Could you check a few things on this model? Use its own coordinates, in mm. A direction names the side the tool comes from. Round coordinates to 2 decimals unless told otherwise and drop trailing zeros. Write each loop counter-clockwise with the first axis right and the second up, starting at its lowest first coordinate (ties: lowest second). Pieces come first, ordered by that corner, then holes. Notation, with made-up numbers: (86.5, -38.75) -> (134.5, -38.75) arc R20 ccw to (134.5, -2.75) -> close; hole circle Ø9 at (62, 89). An arc over 180 degrees is marked (long way). Return JSON: item names as keys, results as strings.
from build123d import *

# Parameters (mm, degrees)
BOSS_EXTRUDE1_DEPTH    = 15
M2_5_CLEARANCE_HOLE1_D = 2.9
M2_5_CLEARANCE_HOLE2_D = 2.9
FILLET1_START          = -15
FILLET1_DEPTH          = 30
FILLET1_START_2        = 4.5
FILLET1_2_OUTLINE_R    = 1.45
FILLET1_2_DEPTH        = 2.5
CUT_EXTRUDE1_START     = -4.5
SKETCH6_R              = 2.75
SKETCH6_R_2            = 2.749999999
CUT_EXTRUDE1_DEPTH     = 10


with BuildPart() as part:
    # Sketch1 → Boss-Extrude1 (new, symmetric)
    with BuildSketch(Plane.XY):
        Polygon((0, 0), (0, -10), (4.5, -10), (4.5, -3.267573076), (86.73, 23.5), (96.73, 23.5), (96.73, 28), (86.016016224, 28), align=None)
    extrude(amount=BOSS_EXTRUDE1_DEPTH, both=True)

    # M2.5 Clearance Hole1 (through all)
    with Locations(Plane(origin=(0, 23.5, 0), x_dir=(-1, 0, 0), z_dir=(0, -1, 0))):
        with Locations((-91.73, -6), (-91.73, 6)):
            Hole(M2_5_CLEARANCE_HOLE1_D / 2)

    # M2.5 Clearance Hole2 (through all)
    with Locations(Plane(origin=(4.5, 0, 0), x_dir=(0, 0, -1), z_dir=(1, 0, 0))):
        with Locations((-10, -6.633786538), (10, -6.633786538)):
            Hole(M2_5_CLEARANCE_HOLE2_D / 2)

    # Fillet1: read off the stored shape, not the designer's step
    # Fillet1 outline → Fillet1 (add)
    with BuildSketch(Plane.XY.offset(FILLET1_START)):
        with BuildLine():
            ThreePointArc((4.5, -10), (6.553657374, -4.444003243), (11.390420445, -1.024598094))
            Line((11.390420445, -1.024598094), (4.5, -3.267573076))
            Line((4.5, -3.267573076), (4.5, -10))
        make_face()
        with BuildLine():
            ThreePointArc((85.221291355, 23.008883997), (86.749601573, 23.376457866), (88.316630614, 23.5))
            Line((88.316630614, 23.5), (86.73, 23.5))
            Line((86.73, 23.5), (85.221291355, 23.008883997))
        make_face()
    extrude(amount=FILLET1_DEPTH)

    # Fillet1 2 outline → Fillet1 2 (cut)
    with BuildSketch(Plane.YZ.offset(FILLET1_START_2)):
        with Locations((-6.633786538, -10)):
            Circle(FILLET1_2_OUTLINE_R)
        with Locations((-6.633786538, 10)):
            Circle(FILLET1_2_OUTLINE_R)
    extrude(amount=FILLET1_2_DEPTH, mode=Mode.SUBTRACT)

    # Sketch6 → Cut-Extrude1 (cut)
    with BuildSketch(Plane.ZY.offset(CUT_EXTRUDE1_START)):
        with Locations(Location((-10, -6.633786538, 0), (0, 0, 270))):
            Circle(SKETCH6_R)
        with Locations(Location((10, -6.633786538, 0), (0, 0, 270))):
            Circle(SKETCH6_R_2)
    extrude(amount=-CUT_EXTRUDE1_DEPTH, mode=Mode.SUBTRACT)


solid = part.part
1) For faces 4 (the face through (92, 23.5, 0)), 5 (the face through (2, -10, 0)), 6 (the face through (5.461, -3.886, 10.121)), which set-ups out of +Z, -Z, +X, -X, +Y, -Y let a thin tool reach every point of the face, with its end or its side?
Return value:
{"face 4": "+Z, -Z, +X, -Y", "face 5": "+Z, -Z, +X, -X, -Y", "face 6": "+X"}
2) I want a section at A-A, the plane x = 91.73. Please give me the cut outline in (y, z).
Return value:
{"outline": "(23.5, -15) -> (28, -15) -> (28, -7.45) -> (23.5, -7.45) -> close; (23.5, -4.55) -> (28, -4.55) -> (28, 4.55) -> (23.5, 4.55) -> close; (23.5, 7.45) -> (28, 7.45) -> (28, 15) -> (23.5, 15) -> close"}
3) I want a section at C-C, the plane z = 2. Please give me the cut outline in (x, y), and give its area (3 significant figures).
Return value:
{"outline": "(0, -10) -> (4.5, -10) arc R10 cw to (11.39, -1.02) -> (85.22, 23.01) arc R10 cw to (88.32, 23.5) -> (96.73, 23.5) -> (96.73, 28) -> (86.02, 28) -> (0, 0) -> close", "area": "492 mm²"}
4) I want a section at D-D, the plane x = 39. Please give me the cut outline in (y, z), and give its area (3 significant figures).
Return value:
{"outline": "(7.96, -15) -> (12.7, -15) -> (12.7, 15) -> (7.96, 15) -> close", "area": "142 mm²"}
5) Will these pins go through, and if not, where does the flat tip stop? pin 1 Ø6 at (y, z) = (-7.5, 11) entering from +X; pin 2 Ø3 at (x, z) = (57.5, 7) entering from -Y; pin 3 Ø2.5 at (y, z) = (-7.5, -9.5) entering from +X.
Return value:
{"pin 1": "x = 6.41", "pin 2": "y = 13.5", "pin 3": "x = 4.5"}
6) Thinking about a two-plate mould opening in Y: for faces 1 (the face through (96.73, 26, 0)), 2 (the face through (2.219, -5.654, 8.931)), 3 (the face through (47.789, 10.824, 0.21)), which applies, pulls with the +Y half, pulls with the -Y half, needs draft (parallel to the pull), parting line crosses it, or undercut?
Return value:
{"face 1": "needs draft", "face 2": "undercut", "face 3": "pulls with the -Y half"}
7) I want a section at B-B, the plane z = -6. Please give me the cut outline in (x, y).
Return value:
{"outline": "(0, -10) -> (4.5, -10) arc R10 cw to (11.39, -1.02) -> (85.22, 23.01) arc R10 cw to (88.32, 23.5) -> (90.28, 23.5) -> (90.28, 28) -> (86.02, 28) -> (0, 0) -> close; (93.18, 23.5) -> (96.73, 23.5) -> (96.73, 28) -> (93.18, 28) -> close"}
8) If I drill on probe 1 along Z at (x, y) = (91, 25); probe 2 along Y at (x, z) = (2, -10); probe 3 along Y at (x, z) = (1.4, -10), over which ranges is the centre line in solid material (lowest first)? Write a range as [from, to].
Return value:
{"probe 1": "[-15, -7.25], [-4.75, 4.75], [7.25, 15]", "probe 2": "[-10, -8.08], [-5.18, 0.65]", "probe 3": "[-10, -8.08], [-5.18, 0.46]"}
